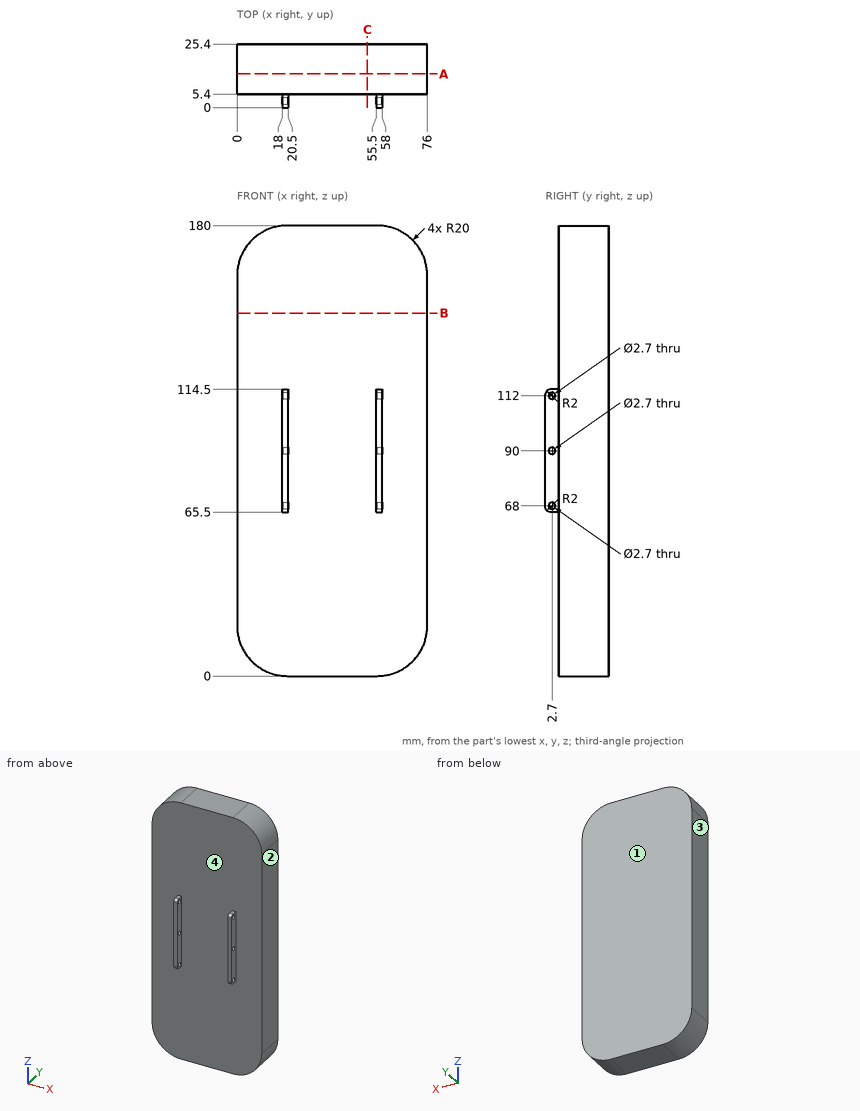
Can you work these out from the drawing? Everything is in mm from the part's minimum corner. Round coordinates to 2 decimals unless told otherwise and drop trailing zeros. Loops run counter-clockwise (first coordinate to the right, second up) from the corner with the lowest first, then second, coordinate; pieces in that order, holes last. Notation, with made-up numbers: (65.5, 52.5) - (108.5, 52.5) arc R7 ccw to (108.5, 64.5) - close; hole circle Ø11 at (27.25, -3.5). An arc over 180 degrees is marked (long way). Answer in a Markdown table with one row per item. Add a question column.
Q1. We'd pull the mould along X, two halves only. Please class the marked faces 1, 2, 3 and 4: pulls with the +X half, pulls with the -X half, needs draft (parallel to the pull), parting line crosses it, or undercut.
Q2. For pin 1 Ø2.5 at (y, z) = (2, 79) entering from -X; pin 2 Ø2 at (x, y) = (19.5, 4) entering from -Z; pin 3 Ø1.2 at (x, y) = (19.5, 4) entering from +Z; pin 4 Ø6 at (y, z) = (3, 84.5) entering from -X, each with a flat end and sliding along its axis, tell me the tip position at first contact or that it passes through.
Q3. I want a section at A-A on y = 13.5. List the corners of the cut face in (x, z) for me.
Q4. I want a section at C-C on x = 52. List the corners of the cut face in (y, z) for me, and give its area (3 significant figures).
Q5. I need wall thicknesses on L1, parallel to Y at x = 19.5, z = 112; L2, parallel to Y at x = 20, z = 158; L3, parallel to Z at x = 62.5, y = 22.75. Which ranges of each line are inside material? Lowest first, please.
Q6. I want a section at B-B on z = 145. List the corners of the cut face in (x, y) for me.
A:
| question | item | result |
|---|---|---|
| 1 | face 1 | needs draft |
| 1 | face 2 | pulls with the +X half |
| 1 | face 3 | pulls with the -X half |
| 1 | face 4 | undercut |
| 2 | pin 1 | x = 18 |
| 2 | pin 2 | z = 65.5 |
| 2 | pin 3 | z = 114.5 |
| 2 | pin 4 | x = 0 |
| 3 | outline | (0, 20) arc R20 ccw to (20, 0) - (56, 0) arc R20 ccw to (76, 20) - (76, 160) arc R20 ccw to (56, 180) - (20, 180) arc R20 ccw to (0, 160) - close |
| 4 | outline | (5.4, 0) - (25.4, 0) - (25.4, 180) - (5.4, 180) - close |
| 4 | area | 3,600 mm^2 |
| 5 | L1 | 0 to 1.35, 4.05 to 25.4 |
| 5 | L2 | 5.4 to 25.4 |
| 5 | L3 | 1.09 to 178.91 |
| 6 | outline | (0, 5.4) - (76, 5.4) - (76, 25.4) - (0, 25.4) - close |
